Here's the drawing with two shaded views (mm, measured from the low corner). I have some questions. Round coordinates to 2 decimals unless told otherwise and drop trailing zeros. Loops run counter-clockwise (first coordinate to the right, second up) from the corner with the lowest first, then second, coordinate; pieces in that order, holes last.
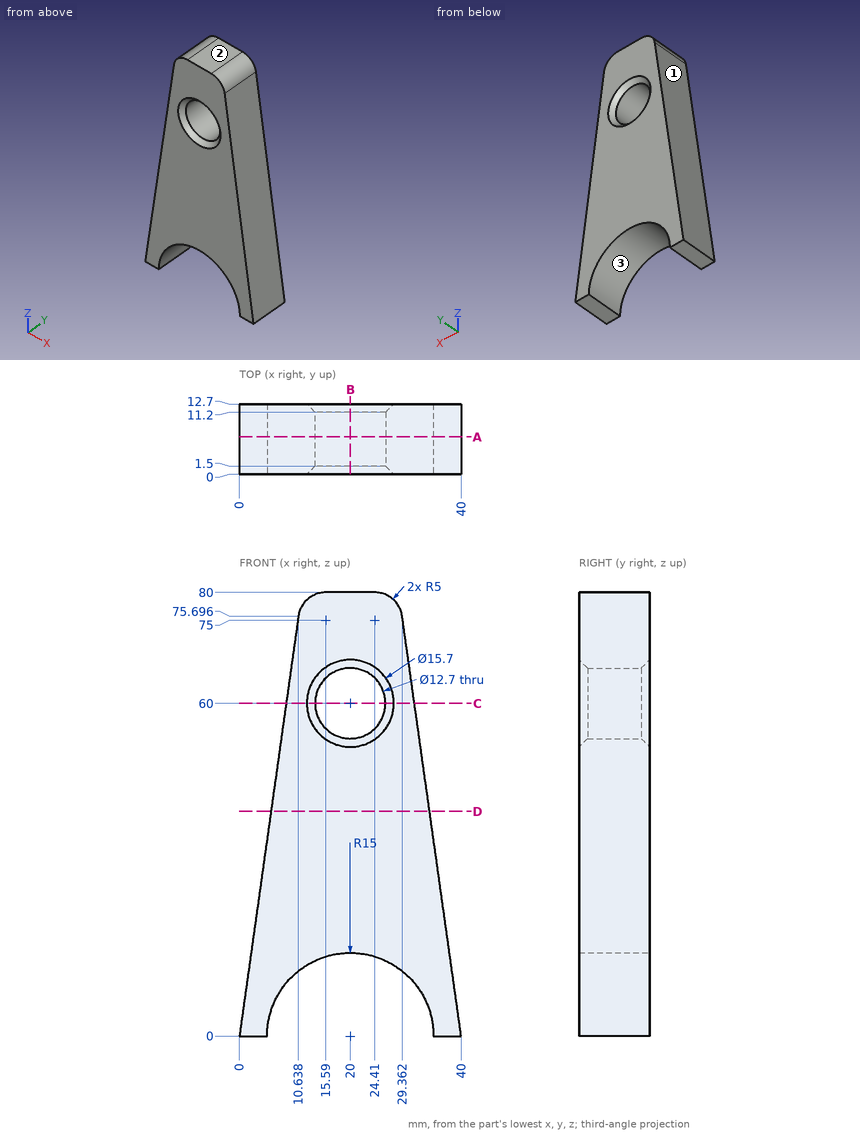
(1) If we mould it in two halves opening along X, with no side actions, what happens to the marked faces 1, 2 and 3? For each: released by +X, released by -X, zero draft, split by the parting line, or undercut.
Worked answers:
face 1: released by -X
face 2: zero draft
face 3: undercut
(2) If I drill on line 1 (Z direction, x = 20, y = 8); line 2 (X direction, y = 3, z = 52.5); line 3 (Z direction, x = 18.5, y = 4.5) (1 decimal), over which ranges is the centre line in solid material (lowest first)?
Worked answers:
line 1: z = 15 to 53.65, 66.35 to 80
line 2: x = 7.38 to 32.62
line 3: z = 14.9 to 53.8, 66.2 to 80
(3) If we section it at A-A, the plane y = 6.75: List the corners of the cut face in (x, z) for me, then the cut area to 3 significant figures.
Worked answers:
outline: (0, 0) - (5, 0) arc R15 cw to (35, 0) - (40, 0) - (29.36, 75.7) arc R5 ccw to (24.41, 80) - (15.59, 80) arc R5 ccw to (10.64, 75.7) - close; hole circle Ø12.7 at (20, 60)
area: 1,810 mm2
(4) If we section it at D-D, the plane z = 40.5: List the corners of the cut face in (x, y) for me, then the cut area to 3 significant figures.
Worked answers:
outline: (5.69, 0) - (34.31, 0) - (34.31, 12.7) - (5.69, 12.7) - close
area: 363 mm2
(5) If we section it at C-C, the plane z = 60: List the corners of the cut face in (x, y) for me.
Worked answers:
outline: (8.43, 0) - (12.15, 0) - (13.65, 1.5) - (13.65, 11.2) - (12.15, 12.7) - (8.43, 12.7) - close; (26.35, 1.5) - (27.85, 0) - (31.57, 0) - (31.57, 12.7) - (27.85, 12.7) - (26.35, 11.2) - close
(6) Will these pins go through, and if not, where does the flat tip stop? P1, Ø2, axis at y = 11, z = 47, coming from the -X side (1 decimal); P2, Ø3, axis at y = 3.5, z = 17.5, coming from the -X side.
Worked answers:
P1: stops at x = 6.5
P2: stops at x = 2.25
(7) If we section it at B-B, the plane x = 20: List the corners of the cut face in (y, z) for me.
Worked answers:
outline: (0, 15) - (12.7, 15) - (12.7, 52.15) - (11.2, 53.65) - (1.5, 53.65) - (0, 52.15) - close; (0, 67.85) - (1.5, 66.35) - (11.2, 66.35) - (12.7, 67.85) - (12.7, 80) - (0, 80) - close
